Solid Edge part; units mm, degrees
sketch "Sketch1" plane through (0, 0, 0) normal (0, 0, 1) x (1, 0, 0)
  line L0 (7.5, 0) -> (7.5, 6.614378)
  line L1 (7.5, 0) -> (7.5, -6.614378)
  arc A0 (7.499989, -6.61439) -> (7.499989, 6.61439) centre (0, 0) cw
extrude "Protrusion1" add sketch "Sketch1" along normal blind 457.2
sketch "Sketch2" plane through (0, 0, 0) normal (0, 0, 1) x (1, 0, 0)
  line L0 (7.5, 0) -> (7.5, 6.614378)
  line L1 (7.5, 0) -> (7.5, -6.614378)
  arc A0 (7.499989, -6.61439) -> (7.499989, 6.61439) centre (0, 0) cw
sketch "Sketch3" plane through (0, 0, 0) normal (1, 0, 0) x (0, 1, 0)
  line L0 (10, 0) -> (8.59, 0)
  line L1 (8.59, 0) -> (10, 1.41)
  line L2 (10, 1.41) -> (10, 0)
sweep "SweptCutout_4" cut profiles "Sketch3" path "Sketch2"
sketch "Sketch4" plane through (0, 0, 0) normal (1, 0, 0) x (0, 1, 0)
  line L0 (10, 457.2) -> (8.59, 457.2)
  line L1 (8.59, 457.2) -> (10, 455.79)
  line L2 (10, 455.79) -> (10, 457.2)
sketch3d "SweptCutout_5 path"
  arc A0 (7.5, -6.614378, 457.2) -> (-10, 0, 457.2) centre (0, 0, 457.2)
  arc A1 (-10, 0, 457.2) -> (7.5, 6.614378, 457.2) centre (0, 0, 457.2)
  line L2 (7.5, 0, 457.2) -> (7.5, 6.614378, 457.2)
sweep "SweptCutout_5" cut profiles "Sketch4" path "SweptCutout_5 path"
sketch "Sketch5" plane through (0, 0, 39) normal (0, 0, 1) x (1, 0, 0)
  line L0 (25.491064, -13.358298) -> (-25.491064, -13.358298)
  line L1 (-25.491064, -13.358298) -> (-25.491064, 13.358298)
  line L2 (-25.491064, 13.358298) -> (25.491064, 13.358298)
  line L3 (25.491064, 13.358298) -> (25.491064, -13.358298)
extrude "ExtrudedCutout_1" cut sketch "Sketch5" along normal blind 433.531277
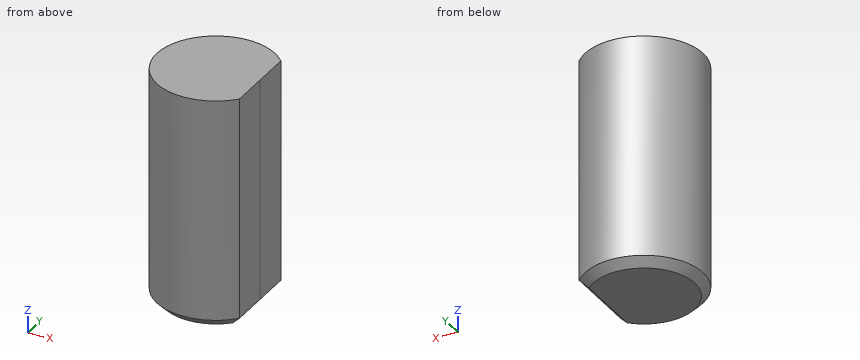
Read the model definition and answer for the solid it produces. Units are mm, in the model's axes. Round coordinates to 2 decimals unless told otherwise and drop trailing zeros. Order: outer loops, then holes, each group sorted by start corner. A loop starts at its lowest first (then second) coordinate and runs counter-clockwise, first axis right, second up.
1) Flat-ended cylindrical pins translate along their axes: pin 1 (1.5 mm diameter, centred on y = -1, z = 11, fed in from -X); pin 2 (6 mm diameter, centred on x = -0.5, z = 20, fed in from +Y). Find the tip coordinate at first contact, or state that the pin passes through.
2) The part is cut by section A-A on z = 33. Write down the section's boundary in (x, y), plus the area to 3 significant figures.
3) Straight lines are drawn through the part: L1, parallel to Y at x = -8.25, z = 27.5; L2, parallel to Y at x = 4.25, z = 22; L3, parallel to X at y = 5.75, z = 27.5. For each, find the intervals that lie inside material, in ascending order.
Resolved:
1. pin 1: stops at x = -10
1. pin 2: stops at y = 10
2. outline: (7.5, -6.61) - (7.5, 6.61) arc R10 ccw (long way) to start
2. area: 291 mm2
3. L1: y = -5.65 to 5.65
3. L2: y = -9.05 to 9.05
3. L3: x = -8.18 to 7.5
